Job drawing, mm, ordinate dimensions from the low corner. One solid piece. Give positions to 0.01 mm unless a question says otherwise; leave off trailing zeros. Order: outer loops, then holes, each group sorted by start corner. A loop starts at its lowest first (then second) coordinate and runs counter-clockwise, first axis right, second up.
1. Slice it at D-D on z = 10. List the corners of the cut face in (x, y) (1 decimal).
2. Probe line 1 (Z direction, x = 8.75, y = 4.25) (1 decimal); line 2 (Y direction, x = 14, z = 22.75); line 3 (X direction, y = 3, z = 24.5) (1 decimal). List the from-to ranges inside material, lowest first.
3. Slice it at A-A on y = 4.75. List the corners of the cut face in (x, z) (1 decimal).
4. Slice it at C-C on x = 16. List the corners of the cut face in (y, z).
5. Mould opens along Z. For the marked faces 1, 2, 3 and 4 say: +Z half, -Z half, draft (parallel to the pull), parting line (faces both ways), or undercut.
6. Drop flat-ended pins along their axis: pin 1 Ø0.9 at (y, z) = (3.5, 24.5) entering from +X; pin 2 Ø3 at (x, y) = (8.43, 2.4) entering from -Z; pin 3 Ø4 at (x, y) = (5, 2.5) entering from +Z. Give the stop position or say it passes through.
7. Slice it at B-B on y = 3. List the corners of the cut face in (x, z) (1 decimal).
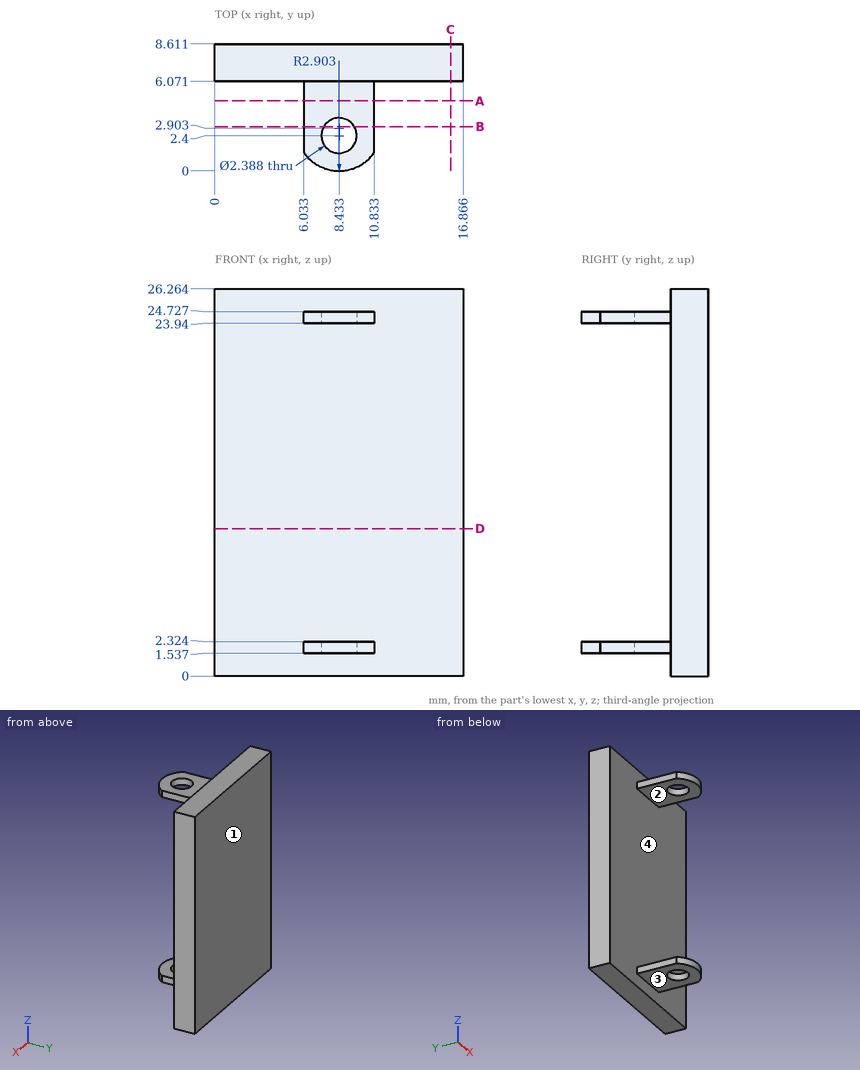
Data:
1. outline: (0, 6.1) - (16.9, 6.1) - (16.9, 8.6) - (0, 8.6) - close
2. line 1: z = 1.5 to 2.3, 23.9 to 24.7
2. line 2: y = 6.07 to 8.61
2. line 3: x = 6 to 7.4, 9.5 to 10.8
3. outline: (6, 1.5) - (10.8, 1.5) - (10.8, 2.3) - (6, 2.3) - close; (6, 23.9) - (10.8, 23.9) - (10.8, 24.7) - (6, 24.7) - close
4. outline: (6.07, 0) - (8.61, 0) - (8.61, 26.26) - (6.07, 26.26) - close
5. face 1: draft
5. face 2: undercut
5. face 3: -Z half
5. face 4: undercut
6. pin 1: stops at x = 10.83
6. pin 2: stops at z = 1.54
6. pin 3: stops at z = 24.73
7. outline: (6, 1.5) - (7.4, 1.5) - (7.4, 2.3) - (6, 2.3) - close; (6, 23.9) - (7.4, 23.9) - (7.4, 24.7) - (6, 24.7) - close; (9.5, 1.5) - (10.8, 1.5) - (10.8, 2.3) - (9.5, 2.3) - close; (9.5, 23.9) - (10.8, 23.9) - (10.8, 24.7) - (9.5, 24.7) - close
